Verification items for the finished model (mm, model axes). Give positions to 0.01 mm unless a question says otherwise; leave off trailing zeros. Order: outer loops, then holes, each group sorted by start corner. A loop starts at its lowest first (then second) coordinate and runs counter-clockwise, first axis right, second up.
Autodesk Inventor part; units mm, degrees
ref_plane "YZ Plane" through (0, 0, 0) normal (1, 0, 0) x (0, 1, 0)
ref_plane "XZ Plane" through (0, 0, 0) normal (0, 1, 0) x (-1, 0, 0)
ref_plane "XY Plane" through (0, 0, 0) normal (0, 0, 1) x (1, 0, 0)
sketch "Sketch1" plane through (0, 0, 0) normal (0, 0, 1) x (1, 0, 0)
  line L0 (-7.8362, 28.532) -> (7.1638, 28.532)
  line L1 (47.1638, -28.0341) -> (-47.8362, -28.0341)
  line L2 (7.1638, 28.532) -> (47.1638, -28.0341)
  line L3 (-7.8362, 28.532) -> (-47.8362, -28.0341)
  line L4 (-7.8362, 28.532) -> (-12.8438, 42.6835)
  line L5 (0.5011, 52.1252) -> (12.1714, 42.6835)
  line L6 (12.1714, 42.6835) -> (7.1638, 28.532)
  line L7 (-47.8362, -28.0341) -> (-79.5254, 61.5206)
  line L8 (-79.5254, 61.5206) -> (-12.8438, 42.6835)
  line L9 (47.1638, -28.0341) -> (78.853, 61.5206)
  line L10 (78.853, 61.5206) -> (12.1714, 42.6835)
  line L11 (78.853, 61.5206) -> (5.0003, 121.2702)
  line L12 (0.5011, 52.1252) -> (5.0003, 121.2702)
  point P0 (0, 0)
  point P1 (-0.3362, 28.532)
  point P2 (-0.3362, -28.0341)
  dimension "d0" = 69.28
  dimension "d1" = 95
  dimension "d2" = 15
  dimension "d3" = 56.566
  dimension "d4" = 69.28
  dimension "d16" = 15.0114
  dimension "d17" = 15.0114
  dimension "d18" = 15.0114
  dimension "d19" = 94.996
  dimension "d20" = 69.2912
  dimension "d21" = 94.996
  dimension "d22" = 69.2912
  dimension "d23" = 94.996
  dimension "d24" = 69.2912
extrude "Extrusion2" add sketch "Sketch1" along normal blind 0.127
sketch "Sketch2" plane through (0, 0, 0.127) normal (0, 0, 1) x (1, 0, 0)
  line L0 (47.1638, -28.0341) -> (78.853, 61.5206)
  line L1 (53.6474, -24.9397) -> (81.9474, 55.0369)
  line L2 (78.0988, 68.6651) -> (12.1448, 122.0244)
  line L3 (5.0003, 121.2702) -> (0.5011, 52.1252)
  line L4 (-0.3988, 116.5308) -> (-4.2384, 57.5244)
  line L5 (-79.5254, 61.5206) -> (-47.8362, -28.0341)
  line L6 (-82.6198, 55.0369) -> (-54.3198, -24.9397)
  line L7 (-42.7562, -33.1141) -> (42.0838, -33.1141)
  line L8 (-7.8362, 28.532) -> (-12.8438, 42.6835)
  line L9 (-12.8438, 42.6835) -> (-79.5254, 61.5206)
  line L10 (78.853, 61.5206) -> (5.0003, 121.2702)
  line L11 (-4.2384, 57.5244) -> (0.8309, 57.1945)
  line L12 (-0.3988, 116.5308) -> (4.6704, 116.2009)
  line L13 (12.1448, 122.0244) -> (8.9496, 118.075)
  line L14 (78.0988, 68.6651) -> (74.9036, 64.7157)
  line L15 (78.853, 61.5206) -> (5.0003, 121.2702)
  line L16 (81.9474, 55.0369) -> (77.1584, 56.7315)
  line L17 (53.6474, -24.9397) -> (48.8584, -23.2451)
  line L18 (42.0838, -33.1141) -> (42.0838, -28.0341)
  line L19 (-47.8362, -28.0341) -> (47.1638, -28.0341)
  line L20 (-42.7562, -33.1141) -> (-42.7562, -28.0341)
  line L21 (-49.5308, -23.2451) -> (-54.3198, -24.9397)
  line L22 (-77.8307, 56.7315) -> (-82.6198, 55.0369)
  line L23 (-12.8438, 42.6835) -> (-79.5254, 61.5206)
  line L24 (-74.6367, 60.1395) -> (-73.2557, 65.0282)
  line L25 (-17.7328, 44.0646) -> (-16.414, 48.9705)
  line L26 (-73.2557, 65.0282) -> (-16.414, 48.9705)
  line L27 (-12.8438, 42.6835) -> (-8.3534, 41.4151)
  line L28 (-7.8362, 28.532) -> (-5.1428, 32.3417)
  line L29 (7.1638, 28.532) -> (-7.8362, 28.532)
  line L30 (-8.3534, 41.4151) -> (-5.1428, 32.3417)
  line L31 (12.1714, 42.6835) -> (7.1638, 28.532)
  line L32 (7.1638, 28.532) -> (4.4702, 32.342)
  line L33 (12.1714, 42.6835) -> (7.6811, 41.4151)
  line L34 (0.5011, 52.1252) -> (0.1988, 47.469)
  line L35 (0.5011, 52.1252) -> (12.1714, 42.6835)
  line L36 (0.1988, 47.469) -> (7.6811, 41.4151)
  line L37 (7.6811, 41.4151) -> (4.4702, 32.342)
  line L38 (4.4702, 32.342) -> (-5.1428, 32.3417)
  line L39 (8.9496, 118.075) -> (74.9036, 64.7157)
  point P0 (0, 0)
  dimension "d34" = 5.08
  dimension "d35" = 5.08
  dimension "d38" = 5.08
  dimension "d39" = 5.08
  dimension "d42" = 5.08
  dimension "d43" = 5.08
  dimension "d46" = 5.08
  dimension "d47" = 5.08
  dimension "d50" = 5.08
  dimension "d51" = 5.08
  dimension "d56" = 5.08
  dimension "d58" = 5.08
  dimension "d64" = 54.74
  dimension "d65" = 3.81
  dimension "d66" = 54.74
  dimension "d67" = 3.81
  dimension "d68" = 54.74
  dimension "d69" = 3.81
  dimension "d70" = 54.74
  dimension "d71" = 3.81
  dimension "d72" = 54.74
  dimension "d73" = 3.81
  dimension "d76" = 5.08
extrude "Extrusion3" add sketch "Sketch2" against normal blind 0.127 contours L0 L16 L1 L17 | L18 L7 L20 L19 | L10 L13 L2 L14 | L21 L6 L22 L5 | L3 L11 L4 L12 | L24 L26 L25 L9 | L35 L33 L36 L34 | L27 L30 L28 L8 | L31 L32 L37 L33 | L28 L38 L32 L29
sketch "Sketch3" plane through (0, 0, 0.127) normal (0, 0, 1) x (1, 0, 0)
  line L0 (8.9496, 118.075) -> (74.9036, 64.7157)
  line L1 (78.853, 61.5206) -> (7.6811, 41.4151)
  line L2 (4.6704, 116.2009) -> (0.8309, 57.1945)
  line L3 (77.1584, 56.7315) -> (48.8584, -23.2451)
  line L4 (47.1638, -28.0341) -> (4.4702, 32.342)
  line L5 (42.0838, -28.0341) -> (-42.7562, -28.0341)
  line L6 (-5.1428, 32.3417) -> (-47.8362, -28.0341)
  line L7 (-49.5308, -23.2451) -> (-77.8307, 56.7315)
  line L8 (-74.6367, 60.1395) -> (-17.7328, 44.0646)
  line L9 (-12.8438, 42.6835) -> (-7.8364, 28.5324)
  line L10 (-7.8364, 28.5324) -> (7.164, 28.5324)
  line L11 (7.164, 28.5324) -> (12.1711, 42.6835)
  line L12 (12.1711, 42.6835) -> (0.5011, 52.1252)
properties part number "Nexus 7 3D hologram frame"
(1) Scan lines: line 1 (Y direction, x = 2, z = 0.05); line 2 (Y direction, x = -14.5, z = 0.05); line 3 (X direction, y = -19.5, z = 0.05). Record each from-to range of solid material in increasing order.
Solved:
line 1: y = -33.11 to 32.34, 46.01 to 116.37
line 2: y = -33.11 to 43.15
line 3: x = -56.24 to 55.57
(2) Section check B-B, the plane y = 84. Enter the section's corners in (x, z), then the cut area to 3 significant figures.
Solved:
outline: (-2.52, 0) - (59.14, 0) - (59.14, 0.13) - (-2.52, 0.13) - close
area: 7.83 mm2
(3) Section check A-A, the plane x = -31.5. Enter the section's corners in (y, z).
Solved:
outline: (-33.11, 0) - (53.23, 0) - (53.23, 0.13) - (-33.11, 0.13) - close
